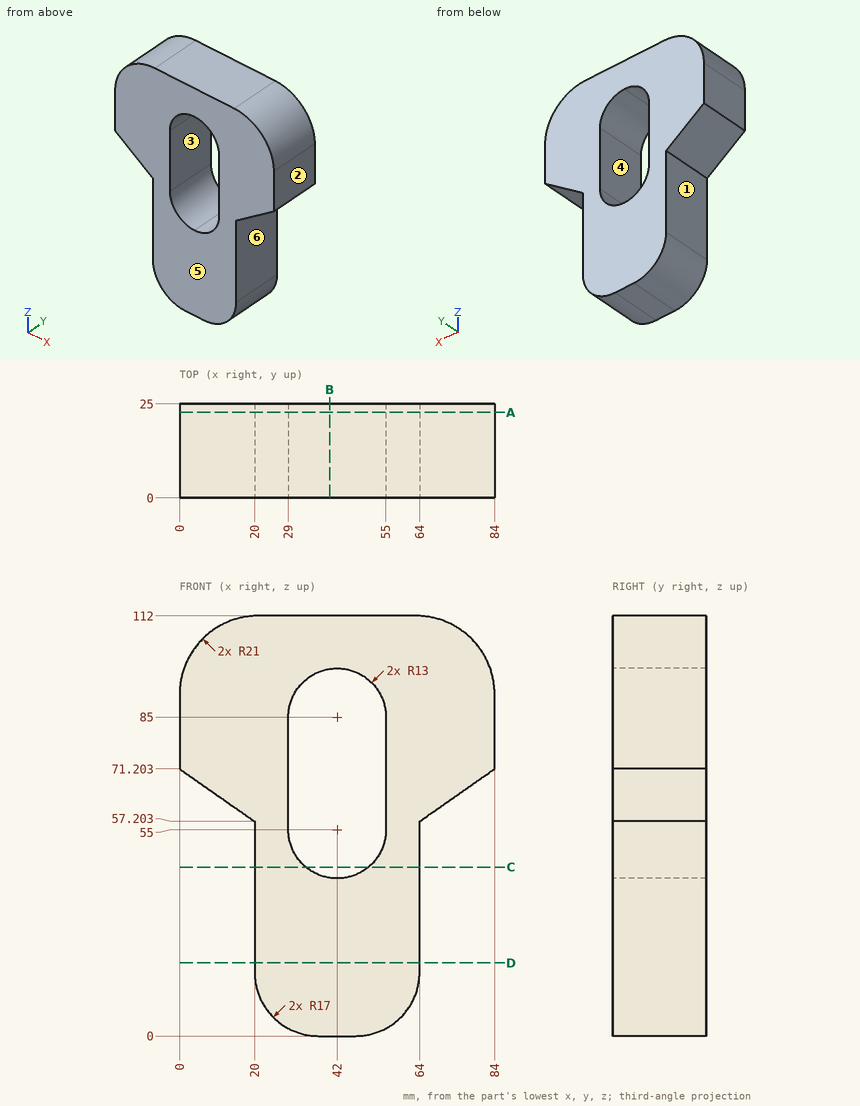
Study the drawing (mm; zero at the part's minimum x, y, z) and answer. A direction names the side the tool comes from. Give positions to 0.01 mm unless a question says otherwise; leave off trailing zeros. Order: outer loops, then holes, each group sorted by start corner. A loop starts at its lowest first (then second) coordinate and runs counter-clockwise, first axis right, second up. Notation, with made-up numbers: (-6.75, 70.5) - (48.25, 70.5) arc R20 cw to (48.25, 107.5) - close; hole circle Ø1 at (-4.75, 70). An arc over 180 degrees is marked (long way). Answer as CSV lines item,"result". Start each with the question number.
Q1. Given pin 1 Ø5 at (x, y) = (9, 4.5) entering from +Z; pin 2 Ø5 at (y, z) = (17.5, 71) entering from +X; pin 3 Ø7.5 at (y, z) = (10, 64) entering from -X; pin 4 Ø1.5 at (y, z) = (19.5, 100.5) entering from -X, each flat-ended and moving along its own axis, determine where each tip first touches the part or whether it passes through.
Q2. The part is cut by section C-C (z = 45). Write down the section's boundary in (x, y), then the cut area to 3 significant figures.
Q3. The part is cut by section B-B (x = 40). Write down the section's boundary in (y, z), then the cut area to 3 significant figures.
Q4. The part is cut by section D-D (z = 19.5). Write down the section's boundary in (x, y), then the cut area to 3 significant figures.
Q5. For the marked faces 5 and 6, determine the directions among +Z, -Z, +X, -X, +Y, -Y from which every point of the face is accessible in a straight line to the end or side of a thin tool.
Q6. The mould has two halves that part along X. Classify the marked faces 1, 2, 3 and 4: +X half, -X half, draft (parallel to the pull), parting line (faces both ways), or undercut.
Q7. Find the intervals of material crossed by L1, parallel to X at y = 12.5, z = 85; L2, parallel to X at y = 13.75, z = 54.5; L3, parallel to X at y = 14.5, z = 21.5, in increasing order. Write a range as [from, to].
Q8. The part is cut by section A-A (y = 22.75). Write down the section's boundary in (x, z), then the cut area to 3 significant figures.
Check result:
1,pin 1,"stops at z = 109.73"
1,pin 2,"stops at x = 84"
1,pin 3,"stops at x = 4.93"
1,pin 4,"stops at x = 1.91"
2,outline,"(20, 0) - (33.69, 0) - (33.69, 25) - (20, 25) - close; (50.31, 0) - (64, 0) - (64, 25) - (50.31, 25) - close"
2,area,"685 mm²"
3,outline,"(0, 0) - (25, 0) - (25, 42.15) - (0, 42.15) - close; (0, 97.85) - (25, 97.85) - (25, 112) - (0, 112) - close"
3,area,"1,410 mm²"
4,outline,"(20, 0) - (64, 0) - (64, 25) - (20, 25) - close"
4,area,"1,100 mm²"
5,face 5,"+Z, -Z, +X, -X, -Y"
5,face 6,"-Z, +X, +Y, -Y"
6,face 1,"-X half"
6,face 2,"+X half"
6,face 3,"undercut"
6,face 4,"undercut"
7,L1,"x = [0, 29], [55, 84]"
7,L2,"x = [20, 29.01], [54.99, 64]"
7,L3,"x = [20, 64]"
8,outline,"(0, 71.2) - (20, 57.2) - (20, 17) arc R17 ccw to (37, 0) - (47, 0) arc R17 ccw to (64, 17) - (64, 57.2) - (84, 71.2) - (84, 91) arc R21 ccw to (63, 112) - (21, 112) arc R21 ccw to (0, 91) - close; hole (29, 55) arc R13 ccw to (42, 42) arc R13 ccw to (55, 55) - (55, 85) arc R13 ccw to (42, 98) arc R13 ccw to (29, 85) - close"
8,area,"5,220 mm²"
